Geometry check sheet. Reference: the model listing, model coordinates, mm. A direction names the side the tool comes from. Give positions to 0.01 mm unless a question says otherwise; leave off trailing zeros. Order: outer loops, then holes, each group sorted by start corner. A loop starts at its lowest first (then second) coordinate and runs counter-clockwise, first axis right, second up. Notation, with made-up numbers: M 11,61 L 33,61 A27 cw 33,84 Z; hole C 47.5,41 d8. An arc over 180 degrees is marked long. Put each result on its own line as item: value. Start each with the question number.
Q1. Section check A-A on z = -38. Record the cut outline in (x, y).
Q2. Section check C-C on x = 43. Record the cut outline in (y, z).
Q3. Material ranges on L1, parallel to Z at x = 19, y = 55; L2, parallel to Y at x = 20.5, z = -7, recorded low to high.
Q4. Mould release check, pull along Y, two halves, no side actions. Record for faces 1 (the cylindrical face through (7.852, 7.504, 5.227)), 2 (the flat face through (32, -9.665, -27)), 3 (the flat face through (6.69, -8, -31)), 4 (the cylindrical face through (10.67, 52.71, 5.23)): +Y half, -Y half, draft (parallel to the pull), parting line (faces both ways), or undercut.
Q5. Section check B-B on y = 19. Record the cut outline in (x, z).
Q6. Go/stop test with flat-tipped pins: pin 1 (8.5 mm diameter, centred on x = 8.19, y = 51.93, fed in from -Z); pin 2 (10 mm diameter, centred on x = 40.5, z = -37.5, fed in from +Y). Record where each tip stops, or that it passes through.
Q7. Access from +Z, -Z, +X, -X, +Y, -Y to the whole of each face (thin tool, end or side, straight path). Record for faces 5 (the flat face through (0, 9, 6)), 6 (the flat face through (32, -6.665, -29)), 7 (the flat face through (9.69, -8, -31)).
Q8. Section check D-D on z = 0. Record the cut outline in (x, y).
```python
from build123d import *

# Parameters (mm, degrees)
EXTRUDE_1_DEPTH     = 65
SKETCH_2_R          = 19.1
SKETCH_2_R_2        = 2.6
CUT_EXTRUDE_1_DEPTH = 65
SKETCH_3_W          = 3
SKETCH_3_H          = 50
CUT_EXTRUDE_2_DEPTH = 10
FILLET_1_R          = 1


with BuildPart() as part:
    # 草图1 → 凸台-拉伸1 (new body)
    with BuildSketch(Plane(origin=(0, 0, 0), x_dir=(0, 0, -1), z_dir=(1, 0, 0))):
        Polygon((-6.706172895, 58.33487067), (-6.706172895, -9.66512933), (61.293827105, -9.66512933), (61.293827105, -6.66512933), (-3.706172895, -6.66512933), (-3.706172895, 58.33487067), align=None)
    extrude(amount=EXTRUDE_1_DEPTH)

    # 草图2 → 切除-拉伸1 (cut)
    with BuildSketch(Plane.XY.offset(6.706172895)):
        with Locations((32.374981494, 29.33487067)):
            Circle(SKETCH_2_R)
        with Locations((8.190858784, 51.925747661)):
            Circle(SKETCH_2_R_2)
        with Locations((55.190858784, 51.925747661)):
            Circle(SKETCH_2_R_2)
        with Locations((8.190858784, 4.925747661)):
            Circle(SKETCH_2_R_2)
        with Locations((55.190858784, 4.925747661)):
            Circle(SKETCH_2_R_2)
    extrude(amount=-CUT_EXTRUDE_1_DEPTH, mode=Mode.SUBTRACT)

    # 草图3 → 切除-拉伸2 (cut)
    with BuildSketch(Plane(origin=(0, -6.66512933, 0), x_dir=(1, 0, 0), z_dir=(0, 1, 0))):
        with Locations((8.19, 31.293827105)):
            Rectangle(SKETCH_3_W, SKETCH_3_H)
        with Locations((56.81, 31.293827105)):
            Rectangle(SKETCH_3_W, SKETCH_3_H)
    extrude(amount=-CUT_EXTRUDE_2_DEPTH, mode=Mode.SUBTRACT)

    # 圆角1
    fillet_1_edges = [part.edges().sort_by_distance(p)[0] for p in [
        (6.69, -8.16512933, -6.293827105),
        (6.69, -8.16512933, -56.293827105),
        (9.69, -8.16512933, -56.293827105),
        (9.69, -8.16512933, -6.293827105),
        (55.31, -8.16512933, -6.293827105),
        (55.31, -8.16512933, -56.293827105),
        (58.31, -8.16512933, -56.293827105),
        (58.31, -8.16512933, -6.293827105),
    ]]
    fillet(fillet_1_edges, radius=FILLET_1_R)


solid = part.part
```
Results found:
1. outline: M 0,-9.67 L 6.69,-9.67 L 6.69,-6.67 L 0,-6.67 Z; M 9.69,-9.67 L 55.31,-9.67 L 55.31,-6.67 L 9.69,-6.67 Z; M 58.31,-9.67 L 65,-9.67 L 65,-6.67 L 58.31,-6.67 Z
2. outline: M -9.67,-61.29 L -6.67,-61.29 L -6.67,3.71 L 13.46,3.71 L 13.46,6.71 L -9.67,6.71 Z; M 45.21,3.71 L 58.33,3.71 L 58.33,6.71 L 45.21,6.71 Z
3. L1: z = 3.71 to 6.71
3. L2: y = -9.67 to -6.67
4. face 1: undercut
4. face 2: -Y half
4. face 3: draft
4. face 4: undercut
5. outline: M 0,3.71 L 16.31,3.71 L 16.31,6.71 L 0,6.71 Z; M 48.44,3.71 L 65,3.71 L 65,6.71 L 48.44,6.71 Z
6. pin 1: stops at z = 3.71
6. pin 2: stops at y = -6.67
7. face 5: +Z, -Z, -X, +Y, -Y
7. face 6: -Z, +X, -X, +Y
7. face 7: +Y, -Y
8. outline: M 0,-9.67 L 65,-9.67 L 65,-6.67 L 0,-6.67 Z
